Source: CAD feature listing. Evaluate the final solid. Frame: model axes, mm. Round coordinates to 2 decimals unless told otherwise and drop trailing zeros. Order: outer loops, then holes, each group sorted by start corner. A loop starts at its lowest first (then second) coordinate and runs counter-clockwise, first axis right, second up. Notation, with made-up numbers: (-37, -9.75) -> (16, -9.75) arc R25 cw to (16, 7.25) -> close; hole circle Ø1 at (-29.5, 78.25). An arc over 180 degrees is marked (long way). Write item = value, one per line. Start each with the question number.
(1) Ray query, line 1 (X direction, y = 0.7, z = 10); line 2 (Z direction, x = 20, y = 0.4); line 3 (Z direction, x = -20, y = 0.65). Return the intervals inside material, ascending.
(2) Cut plane A-A on y = 0.45. Return the cut outline in (x, z), then the cut area to 3 significant figures.
(3) Cut plane B-B on z = 9.5. Return the cut outline in (x, y).
(4) Contact query for flat-ended pins moving along their axis: pin 1 Ø4 at (x, z) = (-20, 10) entering from +Y; pin 2 Ø2.5 at (x, z) = (20, 10) entering from -Y. Output: stop coordinate, or through.
from build123d import *

# Parameters (mm, degrees)
SKETCH1_R           = 1.5
BOSS_EXTRUDE1_DEPTH = 1


with BuildPart() as part:
    # Sketch1 → Boss-Extrude1 (new body)
    with BuildSketch(Plane(origin=(0, 0, 0), x_dir=(1, 0, 0), z_dir=(0, 1, 0))):
        with BuildLine():
            Line((-20, 12), (20, 12))
            ThreePointArc((20, 12), (21.414213562, 11.414213562), (22, 10))
            Line((22, 10), (22, -10))
            ThreePointArc((22, -10), (21.414213562, -11.414213562), (20, -12))
            Line((20, -12), (-20, -12))
            ThreePointArc((-20, -12), (-22, -10), (-20, -8))
            ThreePointArc((-20, -8), (-19.097281882, -7.57092761), (-18.86, -6.6))
            Line((-18.86, -6.6), (-18.86, 6.6))
            ThreePointArc((-18.86, 6.6), (-19.097281882, 7.57092761), (-20, 8))
            ThreePointArc((-20, 8), (-22, 10), (-20, 12))
        make_face()
        with Locations((-20, 10)):
            Circle(SKETCH1_R, mode=Mode.SUBTRACT)
        with Locations((-20, -10)):
            Circle(SKETCH1_R, mode=Mode.SUBTRACT)
        with Locations((20, -10)):
            Circle(SKETCH1_R, mode=Mode.SUBTRACT)
        with Locations((20, 10)):
            Circle(SKETCH1_R, mode=Mode.SUBTRACT)
    extrude(amount=BOSS_EXTRUDE1_DEPTH)


solid = part.part
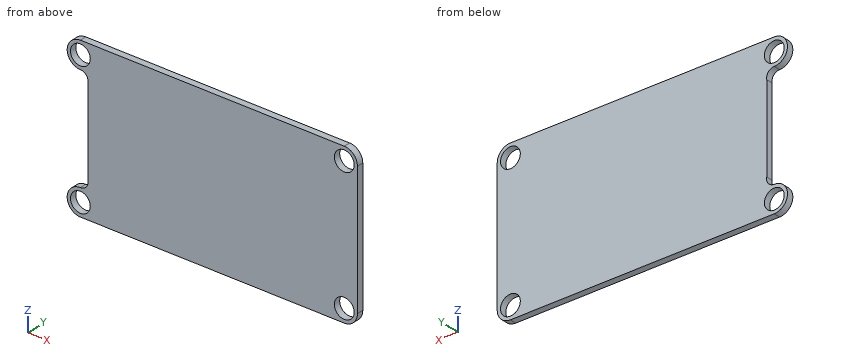
Evaluation:
q1.line_1 = -22 to -21.5, -18.5 to 18.5, 21.5 to 22
q1.line_2 = -12 to -11.5, -8.5 to 8.5, 11.5 to 12
q1.line_3 = -12 to -11.5, -8.5 to -8, 8 to 8.5, 11.5 to 12
q2.outline = (-20, -12) -> (20, -12) arc R2 ccw to (22, -10) -> (22, 10) arc R2 ccw to (20, 12) -> (-20, 12) arc R2 ccw to (-20, 8) arc R1.16 cw to (-18.86, 6.6) -> (-18.86, -6.6) arc R1.16 cw to (-20, -8) arc R2 ccw to start; hole circle Ø3 at (-20, -10); hole circle Ø3 at (-20, 10); hole circle Ø3 at (20, -10); hole circle Ø3 at (20, 10)
q2.area = 973 mm^2
q3.outline = (-21.94, 0) -> (-21.41, 0) -> (-21.41, 1) -> (-21.94, 1) -> close; (-18.59, 0) -> (18.59, 0) -> (18.59, 1) -> (-18.59, 1) -> close; (21.41, 0) -> (22, 0) -> (22, 1) -> (21.41, 1) -> close
q4.pin_1 = 1
q4.pin_2 = through
